from build123d import *

# Parameters (mm, degrees)
BOSS_EXTRU_1_DEPTH           = 15
ENL_V_MAT_EXTRU_1_DEPTH      = 56.901699437
ENL_V_MAT_EXTRU_1_DEPTH_BACK = 56.901699437
ESQUISSE2_W                  = 35
ESQUISSE2_H                  = 10


with BuildPart() as part:
    # Esquisse1 → Boss.-Extru.1 (new body)
    with BuildSketch(Plane(origin=(0, 0, 0), x_dir=(1, 0, 0), z_dir=(0, 1, 0))):
        Polygon((0, 0), (-50, 0), (-50, -5), (-40, -25), (-35, -25), (-35, -5), (0, -5), align=None)
    extrude(amount=BOSS_EXTRU_1_DEPTH)

    # Esquisse2 → Enlèv. mat.-Extru.1 (cut, two sides: drawn at the far end of the back side and taken through both)
    with BuildSketch(Plane.XY.offset(5).offset(-ENL_V_MAT_EXTRU_1_DEPTH_BACK)):
        with Locations((-17.5, 5)):
            Rectangle(ESQUISSE2_W, ESQUISSE2_H)
    extrude(amount=ENL_V_MAT_EXTRU_1_DEPTH + ENL_V_MAT_EXTRU_1_DEPTH_BACK, mode=Mode.SUBTRACT)


solid = part.part
Can you work these out from the model? Positions are in its coordinate system, mm. A direction names the side the tool comes from. Coordinates: 2 decimals unless noted, no trailing zeros. Order: outer loops, then holes, each group sorted by start corner. A loop starts at its lowest first (then second) coordinate and runs counter-clockwise, first axis right, second up. Notation, with made-up numbers: (35, -4.5) - (73, -4.5) arc R25 ccw to (73, 17.5) - close; hole circle Ø11 at (79.5, -24.75). An arc over 180 degrees is marked (long way). Answer as a JSON object with one key per item and string values. Group by question number.
Q1. Imagine slicing it at A-A (y = 9.5). Please give me the cut outline in (x, z), and give its area (3 significant figures).
Q2. Will these pins go through, and if not, where does the flat tip stop? P1, Ø6, axis at x = -24.5, y = 12.5, coming from the +Z side; P2, Ø4, axis at x = -19, z = 3.5, coming from the -Y side; P3, Ø4.5, axis at y = 4.5, z = 8, coming from the +X side.
Q3. Imagine slicing it at C-C (x = -47). Please give me the cut outline in (y, z), and give its area (3 significant figures).
Q4. On a 3-axis mill with a long thin cutter (end or side, diameter ignored), from which of +Z, -Z, +X, -X, +Y, -Y can I reach the whole of each face in a straight line? I mean faces 1 (the face through (-31, 15, 4)), 2 (the face through (-18, 10, 2)), 3 (the face through (-18, 12, 5)). Say none if no direction works.
Q5. Imagine slicing it at D-D (y = 12.5). Please give me the cut outline in (x, z), and give its area (3 significant figures).
Q6. Imagine slicing it at B-B (z = 17.5). Please give me the cut outline in (x, y), and give its area (3 significant figures).
Q7. I need wall thicknesses on line 1 (X direction, y = 9.75, z = 1); line 2 (Y direction, x = -20, z = 2.5); line 3 (X direction, y = 11, z = 18.25) (3 decimals). Which ranges of each line are inside material? Lowest first, please. Write a range as from..to.
Determined:
{
 "1": {"outline": "(-50, 0) - (-35, 0) - (-35, 25) - (-40, 25) - (-50, 5) - close", "area": "275 mm2"},
 "2": {"P1": "stops at z = 5", "P2": "stops at y = 10", "P3": "stops at x = -35"},
 "3": {"outline": "(0, 0) - (15, 0) - (15, 11) - (0, 11) - close", "area": "165 mm2"},
 "4": {"face 1": "+Z, -Z, +X, -X, +Y", "face 2": "+Z, -Z, +X, -Y", "face 3": "+Z, +X, +Y, -Y"},
 "5": {"outline": "(-50, 0) - (0, 0) - (0, 5) - (-35, 5) - (-35, 25) - (-40, 25) - (-50, 5) - close", "area": "450 mm2"},
 "6": {"outline": "(-43.75, 0) - (-35, 0) - (-35, 15) - (-43.75, 15) - close", "area": "131 mm2"},
 "7": {"line 1": "x = -50..-35", "line 2": "y = 10..15", "line 3": "x = -43.375..-35"}
}
